Geometry: final body of the model. Coordinates: model frame, mm. Coordinates: 2 decimals unless noted, no trailing zeros. Write each loop counter-clockwise with the first axis right and the second up, starting at its lowest first coordinate (ties: lowest second). Pieces come first, ordered by that corner, then holes. Notation, with made-up numbers: (6.25, 50.5) - (24.25, 50.5) arc R33 cw to (24.25, 84.5) - close; hole circle Ø6 at (81.25, -6.5). An arc over 180 degrees is marked (long way). Put each result on its own line as item: value.
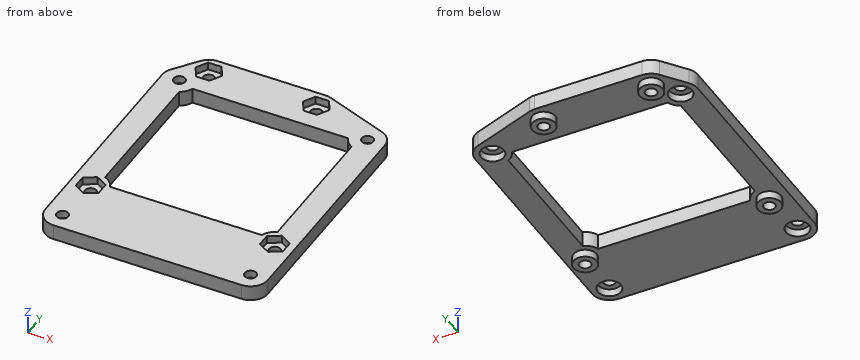
```python
from build123d import *

# Parameters (mm, degrees)
SKETCH_R        = 1.5
PAD_DEPTH       = 2
PAD_DEPTH_BACK  = 2
SKETCH001_R     = 3
SKETCH001_R_2   = 1.5
POCKET_DEPTH    = 2
SKETCH002_R     = 3
SKETCH002_R_2   = 1.5
PAD001_DEPTH    = 4
SKETCH003_R     = 1.5
POCKET001_DEPTH = 5


with BuildPart() as part:
    # Sketch → Pad (new body, two sides)
    with BuildSketch(Plane.XY) as pad_sk:
        with BuildLine():
            ThreePointArc((29, 29), (28.185804, 31.581637), (26.037844, 33.22907))
            Line((9.537844, 39.22907), (26.037844, 33.22907))
            ThreePointArc((9.537844, 39.22907), (8.780763, 39.43175), (8, 39.5))
            Line((-20, 39.5), (8, 39.5))
            ThreePointArc((-20, 39.5), (-22.012461, 39.024922), (-23.6, 37.7))
            Line((-28.1, 31.7), (-23.6, 37.7))
            ThreePointArc((-28.1, 31.7), (-28.769075, 30.423025), (-29, 29))
            Line((-29, 29), (-29, -29))
            ThreePointArc((-29, -29), (-27.68198, -32.181981), (-24.5, -33.5))
            Line((24.5, -33.5), (-24.5, -33.5))
            ThreePointArc((24.5, -33.5), (27.681981, -32.181981), (29, -29))
            Line((29, -29), (29, 29))
        make_face()
        with Locations((-24.5, 29)):
            Circle(SKETCH_R, mode=Mode.SUBTRACT)
        with Locations((-20, 35)):
            Circle(SKETCH_R, mode=Mode.SUBTRACT)
        with Locations((8, 35)):
            Circle(SKETCH_R, mode=Mode.SUBTRACT)
        with Locations((24.5, 29)):
            Circle(SKETCH_R, mode=Mode.SUBTRACT)
        with Locations((24.5, -29)):
            Circle(SKETCH_R, mode=Mode.SUBTRACT)
        with Locations((-24, -16)):
            Circle(SKETCH_R, mode=Mode.SUBTRACT)
        with Locations((-24.5, -29)):
            Circle(SKETCH_R, mode=Mode.SUBTRACT)
        with Locations((24, -16)):
            Circle(SKETCH_R, mode=Mode.SUBTRACT)
        with BuildLine():
            ThreePointArc((-22.460909, 24.988503), (-21.131137, 26.016585), (-20.271383, 27.460909))
            Line((20.271383, 27.460909), (-20.271383, 27.460909))
            ThreePointArc((20.271383, 27.460909), (21.131137, 26.016585), (22.460909, 24.988503))
            Line((22.460909, -11.771383), (22.460909, 24.988503))
            ThreePointArc((22.460909, -11.771383), (20.818019, -12.818019), (19.771383, -14.460909))
            Line((-19.771383, -14.460909), (19.771383, -14.460909))
            ThreePointArc((-19.771383, -14.460909), (-20.818019, -12.818019), (-22.460909, -11.771383))
            Line((-22.460909, 24.988503), (-22.460909, -11.771383))
        make_face(mode=Mode.SUBTRACT)
    extrude(amount=PAD_DEPTH)
    extrude(pad_sk.sketch, amount=-PAD_DEPTH_BACK)

    # Sketch001 → Pocket (cut)
    with BuildSketch(Plane.XY):
        with Locations((-24.5, -29)):
            Circle(SKETCH001_R)
        with Locations((-24.5, -29)):
            Circle(SKETCH001_R_2, mode=Mode.SUBTRACT)
        with Locations((24.5, -29)):
            Circle(SKETCH001_R)
        with Locations((24.5, -29)):
            Circle(SKETCH001_R_2, mode=Mode.SUBTRACT)
        with Locations((24.5, 29)):
            Circle(SKETCH001_R)
        with Locations((24.5, 29)):
            Circle(SKETCH001_R_2, mode=Mode.SUBTRACT)
        with Locations((-24.5, 29)):
            Circle(SKETCH001_R)
        with Locations((-24.5, 29)):
            Circle(SKETCH001_R_2, mode=Mode.SUBTRACT)
    extrude(amount=-POCKET_DEPTH, mode=Mode.SUBTRACT)

    # Sketch002 → Pad001 (join)
    with BuildSketch(Plane.XY):
        with Locations((-20, 35)):
            Circle(SKETCH002_R)
        with Locations((-20, 35)):
            Circle(SKETCH002_R_2, mode=Mode.SUBTRACT)
        with Locations((8, 35)):
            Circle(SKETCH002_R)
        with Locations((8, 35)):
            Circle(SKETCH002_R_2, mode=Mode.SUBTRACT)
        with Locations((24, -16)):
            Circle(SKETCH002_R)
        with Locations((24, -16)):
            Circle(SKETCH002_R_2, mode=Mode.SUBTRACT)
        with Locations((-24, -16)):
            Circle(SKETCH002_R)
        with Locations((-24, -16)):
            Circle(SKETCH002_R_2, mode=Mode.SUBTRACT)
    extrude(amount=-PAD001_DEPTH)

    # Sketch003 → Pocket001 (cut)
    with BuildSketch(Plane.XY):
        Polygon((-16.535898, 35), (-18.267949, 38), (-21.732051, 38), (-23.464102, 35), (-21.732051, 32), (-18.267949, 32), align=None)
        with Locations((-20, 35)):
            Circle(SKETCH003_R, mode=Mode.SUBTRACT)
        Polygon((11.464102, 35), (9.732051, 38), (6.267949, 38), (4.535898, 35), (6.267949, 32), (9.732051, 32), align=None)
        with Locations((8, 35)):
            Circle(SKETCH003_R, mode=Mode.SUBTRACT)
        Polygon((24, -19.464102), (27, -17.732051), (27, -14.267949), (24, -12.535898), (21, -14.267949), (21, -17.732051), align=None)
        with Locations((24, -16)):
            Circle(SKETCH003_R, mode=Mode.SUBTRACT)
        Polygon((-21, -17.732051), (-21, -14.267949), (-24, -12.535898), (-27, -14.267949), (-27, -17.732051), (-24, -19.464102), align=None)
        with Locations((-24, -16)):
            Circle(SKETCH003_R, mode=Mode.SUBTRACT)
    extrude(amount=POCKET001_DEPTH, mode=Mode.SUBTRACT)


solid = part.part
```
1. Section query A-A (z = -3). Return loops of the section in (x, y).
Answer below:
outline: circle Ø6 at (-24, -16); circle Ø6 at (-20, 35); circle Ø6 at (8, 35); circle Ø6 at (24, -16); hole circle Ø3 at (-24, -16); hole circle Ø3 at (-20, 35); hole circle Ø3 at (8, 35); hole circle Ø3 at (24, -16)
2. Pin query (flat end, axial travel): pin 1 Ø4 at (x, y) = (24.5, 29) entering from -Z; pin 2 Ø1.5 at (x, z) = (-6, -2.5) entering from +Y; pin 3 Ø3.5 at (x, y) = (-24, -16) entering from +Z; pin 4 Ø3 at (x, y) = (-5, -14) entering from -Z. Return the tip coordinate at first contact, or that it passes through.
Answer below:
pin 1: stops at z = 0
pin 2: stops at y = 39.5
pin 3: stops at z = 0
pin 4: stops at z = -2
3. Ray query, probe 1 along Y at (x, z) = (6.5, 0.85); probe 2 along X at (y, z) = (-4.5, -0.35); probe 3 along Y at (x, z) = (24.5, 1.55). Return the intervals inside material, ascending. Write a range as from..to.
Answer below:
probe 1: y = -33.5..-14.46, 27.46..32, 38..39.5
probe 2: x = -29..-22.46, 22.46..29
probe 3: y = -33.5..-30.5, -27.5..-19.18, -12.82..27.5, 30.5..33.79
4. Section query B-B (y = -16). Return loops of the section in (x, z), then the cut area to 3 significant figures.
Answer below:
outline: (-29, -2) - (-27, -2) - (-27, -4) - (-25.5, -4) - (-25.5, 0) - (-27, 0) - (-27, 2) - (-29, 2) - close; (-22.5, -4) - (-21, -4) - (-21, -2) - (21, -2) - (21, -4) - (22.5, -4) - (22.5, 0) - (21, 0) - (21, 2) - (-21, 2) - (-21, 0) - (-22.5, 0) - close; (25.5, -4) - (27, -4) - (27, -2) - (29, -2) - (29, 2) - (27, 2) - (27, 0) - (25.5, 0) - close
area: 208 mm²
5. Section query D-D (y = 2.5). Return loops of the section in (x, z), then the cut area to 3 significant figures.
Answer below:
outline: (-29, -2) - (-22.46, -2) - (-22.46, 2) - (-29, 2) - close; (22.46, -2) - (29, -2) - (29, 2) - (22.46, 2) - close
area: 52.3 mm²
6. Section query C-C (x = -11.5). Return loops of the section in (y, z).
Answer below:
outline: (-33.5, -2) - (-14.46, -2) - (-14.46, 2) - (-33.5, 2) - close; (27.46, -2) - (39.5, -2) - (39.5, 2) - (27.46, 2) - close
